```python
from build123d import *

# Parameters (mm, degrees)
F0_W     = 20
F0_H     = 10
F1_DEPTH = 12.5
F2_R     = 2.75
F3_DEPTH = 10
F4_R     = 9.99999
F5_SIZE  = 1


# Not quite as in the source:
# - a fillet or chamfer is up to 0.001 mm smaller than in the source, because OpenCascade refuses the exact size


with BuildPart() as f1:
    # F0 (on Front) → F1 (new body)
    with BuildSketch(Plane.XZ):
        with Locations((10, 5)):
            Rectangle(F0_W, F0_H)
    extrude(amount=F1_DEPTH)

    # F2 (on face) → F3 (cut, through all)
    with BuildSketch(Plane.XY.offset(10)):
        with Locations((10, -6.75)):
            Circle(F2_R)
    extrude(amount=-F3_DEPTH, mode=Mode.SUBTRACT)

    # F4 (radius 10 in the source; OpenCascade refuses exactly that, so slightly less here)
    f4_edges = [f1.edges().sort_by_distance(p)[0] for p in [
        (0, -12.5, 5),
        (20, -12.5, 5),
    ]]
    fillet(f4_edges, radius=F4_R)

    # F5
    f5_edges = [f1.edges().sort_by_distance(p)[0] for p in [
        (17.071071, -9.571071, 0),
        (10.00001, -12.5, 5),
        (20, -2.50001, 5),
        (17.071071, -9.571071, 10),
        (0, 0, 5),
        (10, 0, 0),
        (20, 0, 5),
        (10, 0, 10),
    ]]
    chamfer(f5_edges, length=F5_SIZE)


solid = f1.part
```
Could you check a few things on this model? Use its own coordinates, in mm. Round coordinates to 2 decimals unless told otherwise and drop trailing zeros. One line per question, with ' | ' between items.
Q1. I'm going to push flat-ended pins straight in: pin 1 (1 mm diameter, centred on x = 5.5, z = 4.5, fed in from -Y); pin 2 (4.5 mm diameter, centred on x = 10, y = -6.75, fed in from +Z). Where does each tip first touch, or does it pass through?
Computed values:
pin 1: y = -11.67 | pin 2: through
Q2. We'd pull the mould along X, two halves only. Please class faces 1 (the face through (19.5, -1.8, 9.5)), 2 (the face through (12.54, -7.8, 5.07)), 3 (the face through (3.442, -8.915, 0.174)), 4 (the face through (9.9, -0.5, 0.5)): released by +X, released by -X, zero draft, split by the parting line, or undercut.
Computed values:
face 1: released by +X | face 2: undercut | face 3: released by -X | face 4: zero draft
Q3. If I drill on line 1 (Y direction, x = 10, z = 2.75); line 2 (X direction, y = -7.75, z = 8.25); line 3 (X direction, y = -6, z = 8.75), over which ranges is the centre line in solid material (lowest first)? Write a range as from..to.
Computed values:
line 1: -12.5..-9.5, -4..0 | line 2: 1.49..7.44, 12.56..18.51 | line 3: 0.63..7.35, 12.65..19.37
